Could you check a few things on this model? Use its own coordinates, in mm. A direction names the side the tool comes from. Round coordinates to 2 decimals unless told otherwise and drop trailing zeros. Loops run counter-clockwise (first coordinate to the right, second up) from the corner with the lowest first, then second, coordinate; pieces in that order, holes last. Notation, with made-up numbers: (18.5, 57) -> (50.5, 57) arc R20 ccw to (50.5, 75) -> close; hole circle Ø10 at (-35, 26.25). An arc over 180 degrees is marked (long way). Write each question's results on one line, items separated by ' | '.
from build123d import *

# Parameters (mm, degrees)
SKETCH_1_W      = 48
SKETCH_1_H      = 28
EXTRUDE_1_DEPTH = 37
FILLET_1_R      = 2
SKETCH_2_R      = 2
EXTRUDE_2_DEPTH = 3


with BuildPart() as part:
    # 草图1 → 凸台-拉伸1 (new body)
    with BuildSketch(Plane.XY):
        with Locations((24, 14)):
            Rectangle(SKETCH_1_W, SKETCH_1_H)
    extrude(amount=EXTRUDE_1_DEPTH)

    # 圆角1
    fillet_1_edges = [part.edges().sort_by_distance(p)[0] for p in [
        (48, 14, 37),
        (24, 28, 37),
        (0, 14, 37),
        (24, 28, 0),
        (48, 14, 0),
        (0, 14, 0),
        (0, 28, 18.5),
        (48, 28, 18.5),
        (24, 0, 37),
    ]]
    fillet(fillet_1_edges, radius=FILLET_1_R)

    # 草图2 → 凸台-拉伸2 (add)
    with BuildSketch(Plane.XZ):
        with BuildLine():
            Line((-4, 22.5), (52, 22.5))
            ThreePointArc((52, 22.5), (56, 18.5), (52, 14.5))
            Line((52, 14.5), (-4, 14.5))
            ThreePointArc((-4, 14.5), (-8, 18.5), (-4, 22.5))
        make_face()
        with Locations((-4, 18.5)):
            Circle(SKETCH_2_R, mode=Mode.SUBTRACT)
        with Locations((52, 18.5)):
            Circle(SKETCH_2_R, mode=Mode.SUBTRACT)
    extrude(amount=-EXTRUDE_2_DEPTH)


solid = part.part
1) I want a section at B-B, the plane y = 9.5. Write out the boundary of the cut face in (x, z).
Model answer:
outline: (0, 2) arc R2 ccw to (2, 0) -> (46, 0) arc R2 ccw to (48, 2) -> (48, 35) arc R2 ccw to (46, 37) -> (2, 37) arc R2 ccw to (0, 35) -> close
2) I want a section at A-A, the plane z = 18.5. Write out the boundary of the cut face in (x, y), plus the area to 3 significant figures.
Model answer:
outline: (-8, 0) -> (-6, 0) -> (-6, 3) -> (-8, 3) -> close; (-2, 0) -> (50, 0) -> (50, 3) -> (48, 3) -> (48, 26) arc R2 ccw to (46, 28) -> (2, 28) arc R2 ccw to (0, 26) -> (0, 3) -> (-2, 3) -> close; (54, 0) -> (56, 0) -> (56, 3) -> (54, 3) -> close | area: 1,370 mm2
3) I need wall thicknesses on line 1 (Z direction, x = -4, y = 0.85); line 2 (X direction, y = 22.75, z = 22); line 3 (X direction, y = 15, z = 35.5). Which ranges of each line are inside material? Lowest first, please.
Model answer:
line 1: z = 14.5 to 16.5, 20.5 to 22.5 | line 2: x = 0 to 48 | line 3: x = 0.06 to 47.94
4) I want a section at D-D, the plane z = 13. Write out the boundary of the cut face in (x, y), plus the area to 3 significant figures.
Model answer:
outline: (0, 0) -> (48, 0) -> (48, 26) arc R2 ccw to (46, 28) -> (2, 28) arc R2 ccw to (0, 26) -> close | area: 1,340 mm2
5) If we mould it in two halves opening along X, with no side actions, what happens to faces 6 (the cylindrical face through (47.43, 13.18, 36.4)), 7 (the cylindrical face through (0.57, 13.18, 36.4)), 8 (the cylindrical face through (24.31, 27.43, 36.4)), 9 (the cylindrical face through (51.74, 1.479, 20.483))? For each: released by +X, released by -X, zero draft, split by the parting line, or undercut.
Model answer:
face 6: released by +X | face 7: released by -X | face 8: zero draft | face 9: undercut
6) For faces 1 (the flat face through (-2, 1, 22.5)), 2 (the flat face through (-2, 3, 20)), 3 (the cylindrical face through (24.34, 0.57, 36.4)), 4 (the flat face through (50, 1, 22.5)), 5 (the flat face through (50, 1, 14.5)), which set-ups out of +Z, -Z, +X, -X, +Y, -Y let a thin tool reach every point of the face, with its end or its side?
Model answer:
face 1: +Z, -X, +Y, -Y | face 2: +Z, -Z, -X, +Y | face 3: +Z, +X, -X, -Y | face 4: +Z, +X, +Y, -Y | face 5: -Z, +X, +Y, -Y
7) I'm going to push flat-ended pins straight in: pin 1 (1.5 mm diameter, centred on x = -3, y = 1, fed in from -Z); pin 2 (0.9 mm diameter, centred on x = 50.5, y = 1.5, fed in from +Z); pin 3 (10 mm diameter, centred on y = 10, z = 32.5, fed in from +X); pin 4 (6 mm diameter, centred on x = 18, z = 13, fed in from -Y). Where does each tip first touch, or does it pass through?
Model answer:
pin 1: stops at z = 14.5 | pin 2: stops at z = 22.5 | pin 3: stops at x = 48 | pin 4: stops at y = 0
8) I want a section at C-C, the plane x = -3. Write out the boundary of the cut face in (y, z), plus the area to 3 significant figures.
Model answer:
outline: (0, 14.5) -> (3, 14.5) -> (3, 16.77) -> (0, 16.77) -> close; (0, 20.23) -> (3, 20.23) -> (3, 22.5) -> (0, 22.5) -> close | area: 13.6 mm2
